```python
from build123d import *

# Parameters (mm, degrees)
BOSS_EXTRUDE2_DEPTH                               = 4.7625
SKETCH9_R                                         = 5
CUT_EXTRUDE1_DEPTH                                = 19.581211108
CSK_FOR_M2_5_FLAT_HEAD_MACHINE_SCREW1_D           = 2.9
CSK_FOR_M2_5_FLAT_HEAD_MACHINE_SCREW1_CSINK_D     = 5.5
CSK_FOR_M2_5_FLAT_HEAD_MACHINE_SCREW1_CSINK_ANGLE = 90
CBORE_FOR_2_SOCKET_HEAD_CAP_SCREW1_D              = 2.4384
CBORE_FOR_2_SOCKET_HEAD_CAP_SCREW1_CBORE_D        = 4.7625
CBORE_FOR_2_SOCKET_HEAD_CAP_SCREW1_CBORE_DEPTH    = 2.1844
FILLET1_R                                         = 3.175
CIRPATTERN1_COUNT                                 = 3
SKETCH10_R                                        = 11.176
CUT_EXTRUDE2_DEPTH                                = 1.5875
CHAMFER1_SIZE                                     = 0.508


with BuildPart() as part:
    # Sketch1 → Boss-Extrude2 (new body)
    with BuildSketch(Plane.XY):
        Polygon((12.7, 12.7), (-12.7, 12.7), (0, 0), align=None)
        Polygon((-12.7, 12.7), (-12.7, -12.7), (0, 0), align=None)
        Polygon((0, 0), (-12.7, -12.7), (12.7, -12.7), align=None)
        Polygon((0, 0), (12.7, -12.7), (12.7, 12.7), align=None)
    extrude(amount=BOSS_EXTRUDE2_DEPTH)

    # Sketch9 → Cut-Extrude1 (cut, through all)
    with BuildSketch(Plane.XY.offset(4.7625)):
        Circle(SKETCH9_R)
    extrude(amount=-CUT_EXTRUDE1_DEPTH, mode=Mode.SUBTRACT)

    # CSK for M2.5 Flat Head Machine Screw1 (through all)
    with Locations(Plane(origin=(0, 0, 0), x_dir=(-1, 0, 0), z_dir=(0, 0, -1))):
        with Locations((3.5, 6.062177826)):
            csk_for_m2_5_flat_head_machine_screw1 = CounterSinkHole(CSK_FOR_M2_5_FLAT_HEAD_MACHINE_SCREW1_D / 2, CSK_FOR_M2_5_FLAT_HEAD_MACHINE_SCREW1_CSINK_D / 2, counter_sink_angle=CSK_FOR_M2_5_FLAT_HEAD_MACHINE_SCREW1_CSINK_ANGLE)

    # CBORE for #2 Socket Head Cap Screw1 (through all)
    with Locations(Plane.XY.offset(4.7625)):
        with Locations((0, 0), (-9.779, -9.779), (9.779, -9.779), (-9.779, 9.779)):
            CounterBoreHole(CBORE_FOR_2_SOCKET_HEAD_CAP_SCREW1_D / 2, CBORE_FOR_2_SOCKET_HEAD_CAP_SCREW1_CBORE_D / 2, CBORE_FOR_2_SOCKET_HEAD_CAP_SCREW1_CBORE_DEPTH)

    # Fillet1
    fillet1_edges = [part.edges().sort_by_distance(p)[0] for p in [
        (12.7, 12.7, 2.38125),
        (12.7, -12.7, 2.38125),
        (-12.7, -12.7, 2.38125),
        (-12.7, 12.7, 2.38125),
    ]]
    fillet(fillet1_edges, radius=FILLET1_R)

    # CirPattern1: CSK for M2.5 Flat Head Machine Screw1 ×3 about axis
    cirpattern1_axis = Axis((0, 0, 0), (0, 0, 1))
    for i in range(1, CIRPATTERN1_COUNT):
        add(csk_for_m2_5_flat_head_machine_screw1.rotate(cirpattern1_axis, i * 360 / CIRPATTERN1_COUNT), mode=Mode.SUBTRACT)

    # Sketch10 → Cut-Extrude2 (cut)
    with BuildSketch(Plane.XY.offset(4.7625)):
        Circle(SKETCH10_R)
    extrude(amount=-CUT_EXTRUDE2_DEPTH, mode=Mode.SUBTRACT)

    # Chamfer1
    # the kernel refuses this chamfer: 0.508 mm, written as the material it takes off along each edge
    with BuildSketch(Plane(origin=(0, 0, 4.7625), x_dir=(1, 0, 0), z_dir=(0, -1, 0))) as chamfer1_piece_1:
        Polygon((11.176 + CHAMFER1_SIZE, 0), (11.176, -CHAMFER1_SIZE), (11.176, 0), align=None)
    revolve(axis=Axis((0, 0, 4.7625), (0, 0, 1)), mode=Mode.SUBTRACT)


solid = part.part
```
Source: CAD feature listing. Evaluate the final solid. Frame: model axes, mm. A direction names the side the tool comes from. Round coordinates to 2 decimals unless told otherwise and drop trailing zeros. Write each loop counter-clockwise with the first axis right and the second up, starting at its lowest first coordinate (ties: lowest second). Pieces come first, ordered by that corner, then holes. Notation, with made-up numbers: M 58.25,57.25 L 116.25,57.25 A31 cw 116.25,92.25 Z; hole C -39,48 d11. An arc over 180 degrees is marked long. Answer as a JSON object with one key per item and string values. Group by question number.
(1) Mould query, pull axis Y, two halves, no side actions, for faces 3 (the flat face through (-12.7, 0, 2)), 4 (the flat face through (-8.8, 8.8, 2.578)), 5 (the cylindrical face through (-11.79, -11.75, 2.41)). Classes: +Y half, -Y half, draft (parallel to the pull), parting line (faces both ways), or undercut.
(2) Reachability of faces 1 (the flat face through (12.7, 0, 2)), 2 (the cylindrical face through (-11.669, -11.228, 3.686)) from +Z, -Z, +X, -X, +Y, -Y: full face, straight path, thin tool, end or side. Return the list, or none.
(3) Section query A-A on z = 3.95. State how many separate pieces and enclosed holes the cut face has, then the cut area to 3 significant figures.
(4) Section query C-C on z = 0.3. Output: boundary loops of the cut face in (x, y) (3 decimals).
(5) Ray query, line 1 (Y direction, x = -11.25, z = 4.15); line 2 (Y direction, x = -3, z = 1.65); line 3 (Y direction, x = -10.25, z = 2.75). Return the intervals inside material, ascending. Write a range as [from, to].
(6) First-contact query: pin 1 (2.5 mm diameter, centred on x = -9.5, y = -10.5, fed in from +Z); pin 2 (2.5 mm diameter, centred on x = -3.5, y = -6.06, fed in from -Z); pin 3 (6.5 mm diameter, centred on x = 2, y = -3, fed in from +Z) (3 decimals). Flat tips, straight axial feed; report the tip coordinate or a pass-through.
Computed values:
{
 "1": {"face 3": "draft", "face 4": "undercut", "face 5": "-Y half"},
 "2": {"face 1": "+Z, -Z, +X, +Y, -Y", "face 2": "+Z"},
 "3": {"separate pieces": "1", "enclosed holes": "4", "area": "191 mm^2"},
 "4": {"outline": "M -12.7,-9.525 A3.175 ccw -9.525,-12.7 L 9.525,-12.7 A3.175 ccw 12.7,-9.525 L 12.7,9.525 A3.175 ccw 9.525,12.7 L -9.525,12.7 A3.175 ccw -12.7,9.525 Z; hole C -9.779,-9.779 d2.438; hole C -9.779,9.779 d2.438; hole M -3.457,-3.613 A2.45 ccw long -1.4,-4.8 A5 ccw 4.857,-1.187 A2.45 ccw long 4.857,1.187 A5 ccw -1.4,4.8 A2.45 ccw long -3.457,3.613 A5 ccw Z; hole C 9.779,-9.779 d2.438"},
 "5": {"line 1": "[-12.19, -11.65], [-7.91, 7.91], [11.65, 12.19]", "line 2": "[-12.7, -7.42], [-4.7, -4], [4, 4.7], [7.42, 12.7]", "line 3": "[-12.62, -12.11], [-7.44, 7.44], [12.11, 12.62]"},
 "6": {"pin 1": "z = 2.58", "pin 2": "through", "pin 3": "z = 3.175"}
}
